Could you check a few things on this model? Use its own coordinates, in mm. Face numbers are marked on the shaded views. A direction names the side the tool comes from. Round coordinates to 2 decimals unless told otherwise and drop trailing zeros. Loops run counter-clockwise (first coordinate to the right, second up) from the corner with the lowest first, then second, coordinate; pieces in that order, holes last.
from build123d import *

# Parameters (mm, degrees)
ESQUISSE1_R             = 19
BOSS_EXTRU_1_DEPTH      = 35
ESQUISSE2_R             = 10
BOSS_EXTRU_2_DEPTH      = 5
ESQUISSE3_R             = 3
BOSS_EXTRU_3_DEPTH      = 13
ESQUISSE4_R             = 1.25
ENL_V_MAT_EXTRU_1_DEPTH = 8
ENL_V_MAT_EXTRU_2_DEPTH = 13


with BuildPart() as part:
    # Esquisse1 → Boss.-Extru.1 (new body)
    with BuildSketch(Plane.XY):
        Circle(ESQUISSE1_R)
    extrude(amount=BOSS_EXTRU_1_DEPTH)

    # Esquisse2 → Boss.-Extru.2 (add)
    with BuildSketch(Plane.XY.offset(35)):
        Circle(ESQUISSE2_R)
    extrude(amount=BOSS_EXTRU_2_DEPTH)

    # Esquisse3 → Boss.-Extru.3 (add)
    with BuildSketch(Plane.XY.offset(40)):
        with Locations(Location((0, 0, 0), (0, 0, 180))):
            Circle(ESQUISSE3_R)
    extrude(amount=BOSS_EXTRU_3_DEPTH)

    # Esquisse4 → Enlèv. mat.-Extru.1 (cut)
    with BuildSketch(Plane.XY.offset(35)):
        with Locations((3.239548848, -14.646000248)):
            Circle(ESQUISSE4_R)
        with Locations((9.453296275, -10.326431598)):
            Circle(ESQUISSE4_R)
        with Locations((-13.669600231, -3.023578925)):
            Circle(ESQUISSE4_R)
        with Locations((-14.303582703, 4.517468525)):
            Circle(ESQUISSE4_R)
        with Locations((4.216303956, 13.350010522)):
            Circle(ESQUISSE4_R)
        with Locations((11.064033854, 10.128531723)):
            Circle(ESQUISSE4_R)
    extrude(amount=-ENL_V_MAT_EXTRU_1_DEPTH, mode=Mode.SUBTRACT)

    # Esquisse6 → Enlèv. mat.-Extru.2 (cut)
    with BuildSketch(Plane.XY.offset(53)):
        Polygon((-2.382419019, -1.823205862), (-2.606187886, 1.485861604), (-6.139376272, 1.246937022), (-5.915607406, -2.062130444), align=None)
    extrude(amount=-ENL_V_MAT_EXTRU_2_DEPTH, mode=Mode.SUBTRACT)


solid = part.part
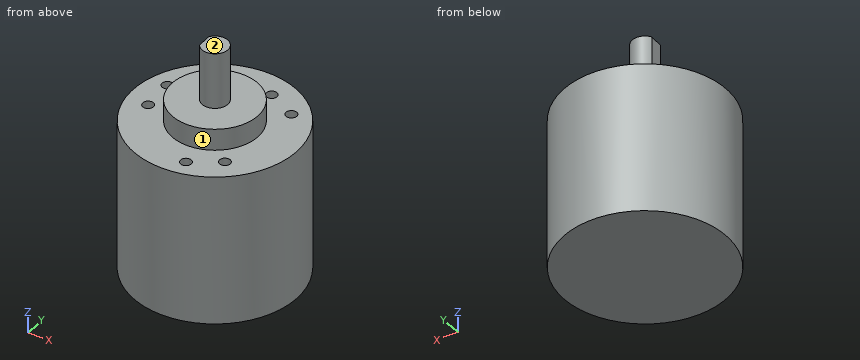
Item 1: For the marked faces 1 and 2, which set-ups out of +Z, -Z, +X, -X, +Y, -Y let a thin tool reach every point of the face, with its end or its side?
Results list:
face 1: +Z
face 2: +Z, +X, -X, +Y, -Y
Item 2: If we section it at D-D, the plane x = 7: Please give me the cut outline in (y, z), then the cut area to 3 significant figures.
Results list:
outline: (-17.66, 0) - (17.66, 0) - (17.66, 35) - (7.14, 35) - (7.14, 40) - (-7.14, 40) - (-7.14, 35) - (-17.66, 35) - close
area: 1,310 mm2
Item 3: If we section it at B-B, the plane z = 38: Please give me the cut outline in (x, y).
Results list:
outline: circle Ø20 at (0, 0)
Item 4: Will these pins go through, and if not, where does the flat tip stop? pin 1 (2 mm diameter, centred on x = 4.22, y = 13.35, fed in from +Z); pin 2 (3 mm diameter, centred on x = 12.5, y = -1, fed in from +Z); pin 3 (8 mm diameter, centred on y = -8.5, z = 43, fed in from -X).
Results list:
pin 1: stops at z = 27
pin 2: stops at z = 35
pin 3: stops at x = -8.11
Item 5: If we section it at A-A, the plane x = 0: Please give me the cut outline in (y, z).
Results list:
outline: (-19, 0) - (19, 0) - (19, 35) - (10, 35) - (10, 40) - (3, 40) - (3, 53) - (-3, 53) - (-3, 40) - (-10, 40) - (-10, 35) - (-19, 35) - close
Item 6: If I drill on line 1 along Y through (x, z) = (0.5, 5); line 2 along Z through (x, y) = (6, 15); line 3 along Z through (x, y) = (9, 2.5), over which ranges is the centre line in solid material (lowest first)?
Results list:
line 1: y = -18.99 to 18.99
line 2: z = 0 to 35
line 3: z = 0 to 40
Item 7: If we section it at C-C, the plane y = 0: Please give me the cut outline in (x, z), then the cut area to 3 significant figures.
Results list:
outline: (-19, 0) - (19, 0) - (19, 35) - (10, 35) - (10, 40) - (3, 40) - (3, 53) - (-2.51, 53) - (-2.51, 40) - (-10, 40) - (-10, 35) - (-19, 35) - close
area: 1,500 mm2
